Source: CAD feature listing. Evaluate the final solid. Frame: model axes, mm. Face numbers are marked on the shaded views. A direction names the side the tool comes from. Round coordinates to 2 decimals unless told otherwise and drop trailing zeros. Loops run counter-clockwise (first coordinate to the right, second up) from the corner with the lowest first, then second, coordinate; pieces in that order, holes last.
Item 1: Section query B-B on x = 109.5. Return loops of the section in (y, z), then the cut area to 3 significant figures.
Item 2: Section query A-A on z = -209.5. Return loops of the section in (x, y), then the cut area to 3 significant figures.
Item 3: Ray query, L1, parallel to Z at x = -160, y = -209.5; L2, parallel to X at y = -174.5, z = -139; L3, parallel to X at y = 92.5, z = 17. Return the intervals inside material, ascending.
Item 4: Access query for the marked faces 1 and 2. Directions: +Z, -Z, +X, -X, +Y, -Y. A direction counts if a zero-diameter tool reaches every point of the face in a straight line with its end or side. Return the directions, or none.
Item 5: Pull-direction query (X, two-part tool) for the marked faces 3, 4 and 5; classes: released by +X, released by -X, zero draft, split by the parting line, or undercut.
```python
from build123d import *

# Parameters (mm, degrees)
F0_W     = 400
F0_H     = 600
F1_DEPTH = 250
F2_W     = 364
F2_H     = 564
F3_DEPTH = 482
F4_W     = 482
F4_H     = 10
F5_DEPTH = 10
F6_W     = 482
F6_H     = 10
F7_DEPTH = 10


with BuildPart() as f1:
    # F0 (on Front) → F1 (new body, symmetric)
    with BuildSketch(Plane.XZ):
        Rectangle(F0_W, F0_H)
    extrude(amount=F1_DEPTH, both=True)

    # F2 (on face) → F3 (cut)
    with BuildSketch(Plane.XZ.offset(250)):
        Rectangle(F2_W, F2_H)
    extrude(amount=-F3_DEPTH, mode=Mode.SUBTRACT)

    # F4 (on face) → F5 (join)
    with BuildSketch(Plane.YZ.offset(-182)):
        with Locations((-9, 146)):
            Rectangle(F4_W, F4_H)
        with Locations((-9, 5)):
            Rectangle(F4_W, F4_H)
        with Locations((-9, -136)):
            Rectangle(F4_W, F4_H)
        with Locations((-9, -277)):
            Rectangle(F4_W, F4_H)
    extrude(amount=F5_DEPTH)

    # F6 (on face) → F7 (join)
    with BuildSketch(Plane(origin=(182, 0, 0), x_dir=(0, -1, 0), z_dir=(-1, 0, 0))):
        with Locations((9, 146)):
            Rectangle(F6_W, F6_H)
        with Locations((9, 5)):
            Rectangle(F6_W, F6_H)
        with Locations((9, -136)):
            Rectangle(F6_W, F6_H)
        with Locations((9, -277)):
            Rectangle(F6_W, F6_H)
    extrude(amount=F7_DEPTH)


solid = f1.part
```
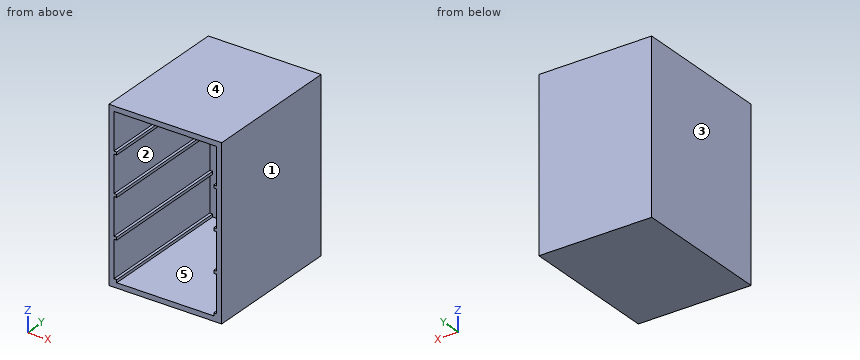
Data:
1. outline: (-250, -300) - (250, -300) - (250, 300) - (-250, 300) - (-250, 282) - (232, 282) - (232, -282) - (-250, -282) - close
1. area: 28,200 mm2
2. outline: (-200, -250) - (-182, -250) - (-182, 232) - (182, 232) - (182, -250) - (200, -250) - (200, 250) - (-200, 250) - close
2. area: 24,600 mm2
3. L1: z = -300 to -282, 282 to 300
3. L2: x = -200 to -172, 172 to 200
3. L3: x = -200 to -182, 182 to 200
4. face 1: +Z, -Z, +X, +Y, -Y
4. face 2: -Y
5. face 3: released by -X
5. face 4: zero draft
5. face 5: undercut
